```python
from build123d import *

# Parameters (mm, degrees)
BASE_FLANGE1_DEPTH = 10
FILLET1_R          = 3
SKETCH5_R          = 1.5
CUT_EXTRUDE1_DEPTH = 17.733200531
SKETCH6_R          = 1.5
CUT_EXTRUDE2_DEPTH = 17.248076809


# Sheet-metal steps are written as plain solids
with BuildPart() as part:
    # Sketch2 → Base-Flange1 (new, symmetric)
    with BuildSketch(Plane.XY):
        with BuildLine():
            Line((0, 8), (0, 2.75))
            ThreePointArc((0, 2.75), (-0.805456352, 0.805456352), (-2.75, 0))
            Line((-2.75, 0), (-12, 0))
            Line((-12, 0), (-12, 2))
            Line((-12, 2), (-2.75, 2))
            ThreePointArc((-2.75, 2), (-2.219669914, 2.219669914), (-2, 2.75))
            Line((-2, 2.75), (-2, 8))
            Line((-2, 8), (0, 8))
        make_face()
    extrude(amount=BASE_FLANGE1_DEPTH, both=True)

    # Fillet1
    fillet1_edges = [part.edges().sort_by_distance(p)[0] for p in [
        (-1, 8, 10),
        (-1, 8, -10),
        (-12, 1, 10),
        (-12, 1, -10),
    ]]
    fillet(fillet1_edges, radius=FILLET1_R)

    # Sketch5 → Cut-Extrude1 (cut, through all)
    with BuildSketch(Plane(origin=(0, 2, 0), x_dir=(1, 0, 0), z_dir=(0, 1, 0))):
        with Locations(Location((-9.28, 6, 0), (0, 0, 270))):
            Circle(SKETCH5_R)
        with Locations(Location((-9.28, -6, 0), (0, 0, 270))):
            Circle(SKETCH5_R)
    extrude(amount=-CUT_EXTRUDE1_DEPTH, mode=Mode.SUBTRACT)

    # Sketch6 → Cut-Extrude2 (cut, through all)
    with BuildSketch(Plane.ZY.offset(2)):
        with Locations(Location((0, 6, 0), (0, 0, 270))):
            Circle(SKETCH6_R)
    extrude(amount=-CUT_EXTRUDE2_DEPTH, mode=Mode.SUBTRACT)


solid = part.part
```
The model under review builds one solid part; all positions refer to its coordinate system, in mm. A direction names the side the tool comes from. Round coordinates to 2 decimals unless told otherwise and drop trailing zeros. Order: outer loops, then holes, each group sorted by start corner. A loop starts at its lowest first (then second) coordinate and runs counter-clockwise, first axis right, second up.
(1) Mouldability with a two-part tool opening along Y and no side actions: class faces 3 (the face through (-1.01, 7.5, 0.07)), 4 (the face through (-0.99, 7.1, 9.14)), 5 (the face through (-0.78, 0.83, 0.14)), 6 (the face through (-12, 1, 0)) as released by +Y, released by -Y, zero draft, split by the parting line, or undercut.
Working result:
face 3: undercut
face 4: released by +Y
face 5: released by -Y
face 6: zero draft
(2) Tool access review of faces 1 (the face through (-7, 2, 0)), 2 (the face through (-0.99, 7.1, -9.14)): name each direction out of +Z, -Z, +X, -X, +Y, -Y from which nothing blocks a thin tool from reaching the whole face with its end or side.
Working result:
face 1: +Z, -Z, -X, +Y
face 2: -Z, +X, -X, +Y
(3) Take a section at D-D, the plane y = 1. State the section outline as (x, z) points.
Working result:
outline: (-12, -7) arc R3 ccw to (-9, -10) - (-0.63, -10) - (-0.63, 10) - (-9, 10) arc R3 ccw to (-12, 7) - close; hole circle Ø3 at (-9.28, -6); hole circle Ø3 at (-9.28, 6)
(4) Wall thickness on L1, parallel to X at y = 5, z = -1.5; L2, parallel to Y at x = -4.25, z = -7; L3, parallel to X at y = 1.5, z = -6: over which ranges is each line inside the solid? List them lowest first.
Working result:
L1: x = -2 to 0
L2: y = 0 to 2
L3: x = -12 to -10.78, -7.78 to -0.3
(5) For P1, Ø2, axis at x = -3.5, z = -2.5, coming from the +Y side, flat-tipped, find the tip position at first contact; note if it passes through.
Working result:
P1: stops at y = 2.04
(6) Take a section at C-C, the plane x = -9.28. State the section outline as (y, z) points, plus the area to 3 significant figures.
Working result:
outline: (0, -9.99) - (2, -9.99) - (2, -7.5) - (0, -7.5) - close; (0, -4.5) - (2, -4.5) - (2, 4.5) - (0, 4.5) - close; (0, 7.5) - (2, 7.5) - (2, 9.99) - (0, 9.99) - close
area: 27.9 mm2
(7) Take a section at A-A, the plane z = 6. State the section outline as (x, y) points, plus the area to 3 significant figures.
Working result:
outline: (-12, 0) - (-10.78, 0) - (-10.78, 2) - (-12, 2) - close; (-7.78, 0) - (-2.75, 0) arc R2.75 ccw to (0, 2.75) - (0, 8) - (-2, 8) - (-2, 2.75) arc R0.75 cw to (-2.75, 2) - (-7.78, 2) - close
area: 28.5 mm2
(8) Take a section at B-B, the plane y = 7. State the section outline as (x, z) points, plus the area to 3 significant figures.
Working result:
outline: (-2, -9.24) - (0, -9.24) - (0, -1.12) - (-2, -1.12) - close; (-2, 1.12) - (0, 1.12) - (0, 9.24) - (-2, 9.24) - close
area: 32.5 mm2
